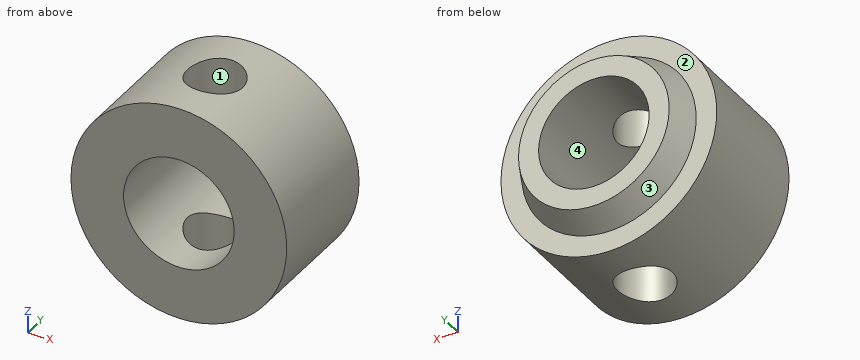
```python
from build123d import *

# Parameters (mm, degrees)
M2_5X0_45_TAPPED_HOLE1_D = 2.05


with BuildPart() as part:
    # Sketch2 → Revolve1 (revolve)
    with BuildSketch(Plane.XY):
        Polygon((2.05, 5.461), (2.05, 0), (4.0005, 0), (4.0005, 4.5212), (3.2385, 4.5212), (2.794, 5.461), align=None)
    revolve(axis=Axis((0, 0, 0), (0, 1, 0)))

    # M2.5x0.45 Tapped Hole1 (through all)
    with Locations(Plane(origin=(0, 2.2606, 4.0005), x_dir=(1, 0, 0), z_dir=(0, 0, 1))):
        with Locations((0, 0)):
            Hole(M2_5X0_45_TAPPED_HOLE1_D / 2)


solid = part.part
```
CAD build for the part. Positions are in the model's coordinates, mm. Face numbers are marked on the shaded views. Coordinates: 2 decimals unless noted, no trailing zeros. Write each loop counter-clockwise with the first axis right and the second up, starting at its lowest first coordinate (ties: lowest second). Pieces come first, ordered by that corner, then holes.
(1) Flat gauge pin, fed straight in: pin 1 (1 mm diameter, centred on y = 4.5, z = -1, fed in from +X). Where does the tip first touch, or does it go through?
(2) Cut at B-B, the plane z = 0. List the corners of the cut face in (x, y).
(3) Cut at C-C, the plane y = 1.45. List the corners of the cut face in (x, z), and give its area (3 significant figures).
(4) Cut at A-A, the plane x = 0. List the corners of the cut face in (y, z).
(5) Two-plate mould, pull along X, no slides. Class the marked faces 1, 2, 3 and 4: +X half, -X half, draft (parallel to the pull), parting line (faces both ways), or undercut.
(6) Cut at D-D, the plane z = 3.75. List the corners of the cut face in (x, y) (3 decimals), and give its area (3 significant figures).
(7) Drill centre lines: probe 1 along X at (y, z) = (1.8, 0); probe 2 along Y at (x, z) = (0, 2.6); probe 3 along Y at (x, z) = (0, 3.3). Where is each one in solid material? Low to high.
Geometry says:
1. pin 1: stops at x = 3.97
2. outline: (-4, 0) - (-2.05, 0) - (-2.05, 5.46) - (-2.79, 5.46) - (-3.24, 4.52) - (-4, 4.52) - close; (2.05, 0) - (4, 0) - (4, 4.52) - (3.24, 4.52) - (2.79, 5.46) - (2.05, 5.46) - close
3. outline: (-0.63, -3.95) - (-0.63, -1.95) arc R2.05 cw to (-0.63, 1.95) - (-0.63, 3.95) arc R4 ccw to start; (0.63, -3.95) arc R4 ccw to (0.63, 3.95) - (0.63, 1.95) arc R2.05 cw to (0.63, -1.95) - close
3. area: 32.1 mm2
4. outline: (0, -4) - (1.24, -4) - (1.24, -2.05) - (0, -2.05) - close; (0, 2.05) - (1.24, 2.05) - (1.24, 4) - (0, 4) - close; (3.29, -4) - (4.52, -4) - (4.52, -3.24) - (5.46, -2.79) - (5.46, -2.05) - (3.29, -2.05) - close; (3.29, 2.05) - (5.46, 2.05) - (5.46, 2.79) - (4.52, 3.24) - (4.52, 4) - (3.29, 4) - close
5. face 1: undercut
5. face 2: draft
5. face 3: parting line
5. face 4: undercut
6. outline: (-1.393, 0) - (1.393, 0) - (1.393, 4.521) - (-1.393, 4.521) - close; hole circle Ø2.05 at (0, 2.261)
6. area: 9.30 mm2
7. probe 1: x = -4 to -2.05, 2.05 to 4
7. probe 2: y = 0 to 1.24, 3.29 to 5.46
7. probe 3: y = 0 to 1.24, 3.29 to 4.52
